from build123d import *

# Parameters (mm, degrees)
SKETCH1_W           = 30
SKETCH1_H           = 120
BOSS_EXTRUDE1_DEPTH = 25
SKETCH2_W           = 10
SKETCH2_H           = 100
CUT_EXTRUDE1_DEPTH  = 26
SKETCH3_W           = 160
SKETCH3_H           = 12.5
SKETCH4_W           = 160
SKETCH4_H           = 12.5
FILLET1_R           = 3
FILLET2_R           = 10
SKETCH5_R           = 12.5
CUT_EXTRUDE2_DEPTH  = 3
SKETCH6_R           = 12.5
CUT_EXTRUDE3_DEPTH  = 3


with BuildPart() as part:
    # Sketch1 → Boss-Extrude1 (new body)
    with BuildSketch(Plane.XY.offset(25)):
        Rectangle(SKETCH1_W, SKETCH1_H)
    extrude(amount=-BOSS_EXTRUDE1_DEPTH)

    # Sketch2 → Cut-Extrude1 (cut, through all)
    with BuildSketch(Plane(origin=(0, 0, 0), x_dir=(-1, 0, 0), z_dir=(0, 0, -1))):
        Rectangle(SKETCH2_W, SKETCH2_H)
    extrude(amount=-CUT_EXTRUDE1_DEPTH, mode=Mode.SUBTRACT)

    # Sketch3 → Revolve1 (revolve)
    with BuildSketch(Plane.XY.offset(12.5)):
        with Locations((-95, 6.25)):
            Rectangle(SKETCH3_W, SKETCH3_H)
    revolve(axis=Axis((-175, 0, 12.5), (1, 0, 0)))

    # Sketch4 → Revolve2 (revolve)
    with BuildSketch(Plane(origin=(0, 0, 12.5), x_dir=(-1, 0, 0), z_dir=(0, 0, -1))):
        with Locations((-95, 6.25)):
            Rectangle(SKETCH4_W, SKETCH4_H)
    revolve(axis=Axis((175, 0, 12.5), (-1, 0, 0)))

    # Fillet1
    fillet1_edges = [part.edges().sort_by_distance(p)[0] for p in [
        (-5, -50, 12.5),
        (5, -50, 12.5),
        (5, 50, 12.5),
        (-5, 50, 12.5),
    ]]
    fillet(fillet1_edges, radius=FILLET1_R)

    # Fillet2
    fillet2_edges = [part.edges().sort_by_distance(p)[0] for p in [
        (-15, 60, 12.5),
        (15, 60, 12.5),
        (15, -60, 12.5),
        (-15, -60, 12.5),
    ]]
    fillet(fillet2_edges, radius=FILLET2_R)

    # Sketch5 → Cut-Extrude2 (cut)
    with BuildSketch(Plane(origin=(175, 0, 0), x_dir=(0, 0, -1), z_dir=(1, 0, 0))):
        with Locations((-12.5, 0)):
            Circle(SKETCH5_R)
    extrude(amount=-CUT_EXTRUDE2_DEPTH, mode=Mode.SUBTRACT)

    # Sketch6 → Cut-Extrude3 (cut)
    with BuildSketch(Plane.ZY.offset(175)):
        with Locations((12.5, 0)):
            Circle(SKETCH6_R)
    extrude(amount=-CUT_EXTRUDE3_DEPTH, mode=Mode.SUBTRACT)


solid = part.part
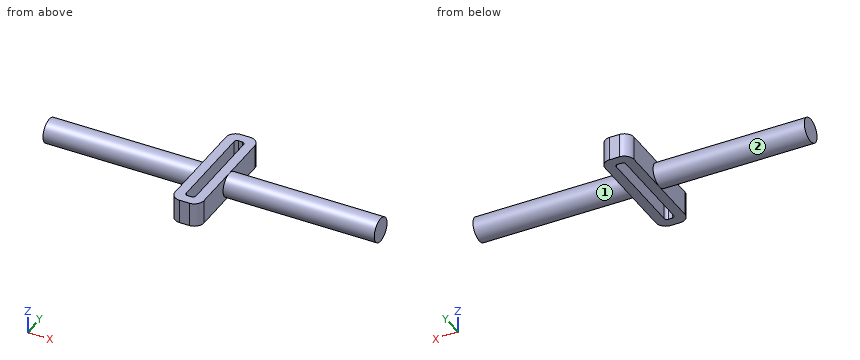
The listing builds one solid part. Answer for the finished solid, in the listing's coordinates (mm). Face numbers are marked on the shaded views. A direction names the side the tool comes from. Give positions to 0.01 mm unless a question says otherwise; leave off trailing zeros. Write each loop counter-clockwise with the first axis right and the second up, starting at its lowest first coordinate (ties: lowest second). Pieces come first, ordered by that corner, then holes.
Item 1: Section D-D, the plane y = 53 is taken. Write down the section's boundary in (x, z).
Item 2: Which of the six approach directions +Z, -Z, +X, -X, +Y, -Y give full straight-line access (tool end or side, diameter ignored) to the marked faces 1 and 2?
Item 3: Section B-B, the plane z = 12.5 is taken. Write down the section's boundary in (x, y).
Item 4: Section A-A, the plane y = -21.5 is taken. Write down the section's boundary in (x, z), plus the area to 3 significant figures.
Item 5: Section C-C, the plane x = -30.5 is taken. Write down the section's boundary in (y, z).
Item 6: Find the intervals of material crossed by line 1 along X through (y, z) = (-36.5, 6.5); line 2 along Y through (x, z) = (2.5, 13.25); line 3 along Y through (x, z) = (60, 13.25), in increasing order.
Item 7: Flat-ended cylindrical pins translate along their axes: P1, Ø4, axis at x = 109.5, z = 6.5, coming from the -Y side; P2, Ø12.5, axis at y = 19, z = 7, coming from the -X side; P3, Ø4, axis at x = -64, z = 5, coming from the +Y side (3 decimals). Find the tip coordinate at first contact, or state that the pin passes through.
Completed:
1. outline: (-14.54, 0) - (14.54, 0) - (14.54, 25) - (-14.54, 25) - close
2. face 1: +X
2. face 2: -X
3. outline: (-172, -12.5) - (-15, -12.5) - (-15, -50) arc R10 ccw to (-5, -60) - (5, -60) arc R10 ccw to (15, -50) - (15, -12.5) - (172, -12.5) - (172, 12.5) - (15, 12.5) - (15, 50) arc R10 ccw to (5, 60) - (-5, 60) arc R10 ccw to (-15, 50) - (-15, 12.5) - (-172, 12.5) - close; hole (-5, -47) arc R3 ccw to (-2, -50) - (2, -50) arc R3 ccw to (5, -47) - (5, 47) arc R3 ccw to (2, 50) - (-2, 50) arc R3 ccw to (-5, 47) - close
4. outline: (-15, 0) - (-5, 0) - (-5, 25) - (-15, 25) - close; (5, 0) - (15, 0) - (15, 25) - (5, 25) - close
4. area: 500 mm2
5. outline: circle Ø25 at (0, 12.5)
6. line 1: x = -15 to -5, 5 to 15
6. line 2: y = -60 to -49.96, 49.96 to 60
6. line 3: y = -12.48 to 12.48
7. P1: stops at y = -11.84
7. P2: stops at x = -15
7. P3: stops at y = 11.225
